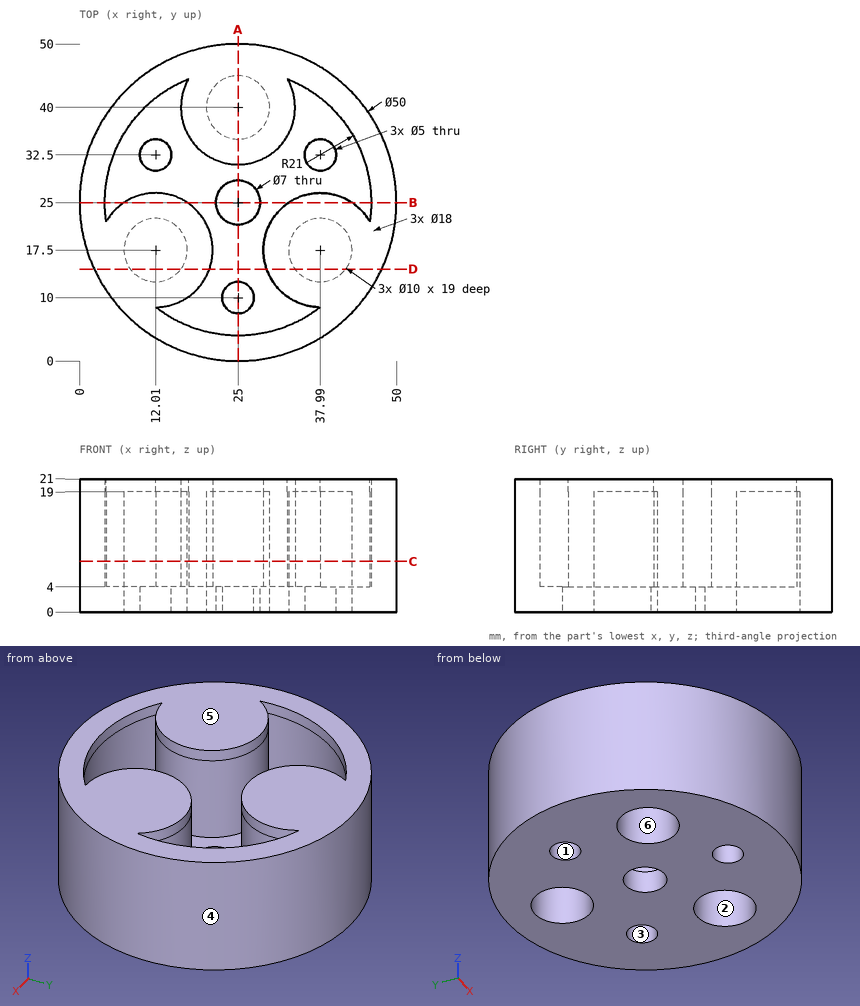
Check sheet for the drawn part. Datum: minimum x, y, z corner. Units: mm. A direction names the side the tool comes from. Coordinates: 2 decimals unless noted, no trailing zeros. Loops run counter-clockwise (first coordinate to the right, second up) from the corner with the lowest first, then second, coordinate; pieces in that order, holes last. Notation, with made-up numbers: (21, 38) -> (56, 38) arc R22 cw to (56, 55) -> close; hole circle Ø10 at (61, -6.75). An arc over 180 degrees is marked (long way). Answer in a Markdown table with one row per item.
1) Section check A-A (x = 25). Record the cut outline in (y, z).
The answers:
| item | result |
|---|---|
| outline | (0, 0) -> (7.5, 0) -> (7.5, 4) -> (4, 4) -> (4, 21) -> (0, 21) -> close; (12.5, 0) -> (21.5, 0) -> (21.5, 4) -> (12.5, 4) -> close; (28.5, 0) -> (35, 0) -> (35, 19) -> (45, 19) -> (45, 0) -> (50, 0) -> (50, 21) -> (31, 21) -> (31, 4) -> (28.5, 4) -> close |
2) Section check C-C (z = 8). Record the cut outline in (x, y) (1 decimal).
The answers:
| item | result |
|---|---|
| outline | circle Ø50 at (25, 25); hole (4.2, 22) arc R9 cw (long way) to (12, 8.5) arc R21 ccw to (38, 8.5) arc R9 cw (long way) to (45.8, 22) arc R21 ccw to (32.8, 44.5) arc R9 cw (long way) to (17.2, 44.5) arc R21 ccw to start; hole circle Ø10 at (12, 17.5); hole circle Ø10 at (25, 40); hole circle Ø10 at (38, 17.5) |
3) Access from +Z, -Z, +X, -X, +Y, -Y to the whole of each face (thin tool, end or side, straight path). Record for the marked faces 1 and 2.
The answers:
| item | result |
|---|---|
| face 1 | +Z, -Z |
| face 2 | -Z |
4) Draft check along X on the marked faces 3, 4, 5 and 6. Enter one of: released by +X, released by -X, zero draft, split by the parting line, or undercut.
The answers:
| item | result |
|---|---|
| face 3 | undercut |
| face 4 | split by the parting line |
| face 5 | zero draft |
| face 6 | undercut |
5) Scan lines: line 1 along Y through (x, z) = (25, 1); line 2 along X through (y, z) = (32.5, 2.5); line 3 along Y through (x, z) = (30.5, 16.75) (1 decimal). Record each from-to range of solid material in increasing order. Write a range as from..to.
The answers:
| item | result |
|---|---|
| line 1 | y = 0..7.5, 12.5..21.5, 28.5..35, 45..50 |
| line 2 | x = 1.15..9.51, 14.51..35.49, 40.49..48.85 |
| line 3 | y = 0.6..4.7, 12.5..22.5, 32.9..49.4 |
6) Section check B-B (y = 25). Record the cut outline in (x, z) (1 decimal), and give its area (3 significant figures).
The answers:
| item | result |
|---|---|
| outline | (0, 0) -> (21.5, 0) -> (21.5, 4) -> (17, 4) -> (17, 21) -> (7, 21) -> (7, 4) -> (4, 4) -> (4, 21) -> (0, 21) -> close; (28.5, 0) -> (50, 0) -> (50, 21) -> (46, 21) -> (46, 4) -> (43, 4) -> (43, 21) -> (33, 21) -> (33, 4) -> (28.5, 4) -> close |
| area | 646 mm2 |
7) Section check D-D (y = 14.5). Record the cut outline in (x, z) (1 decimal), and give its area (3 significant figures).
The answers:
| item | result |
|---|---|
| outline | (2.3, 0) -> (8, 0) -> (8, 19) -> (16, 19) -> (16, 0) -> (34, 0) -> (34, 19) -> (42, 19) -> (42, 0) -> (47.7, 0) -> (47.7, 21) -> (29.5, 21) -> (29.5, 4) -> (20.5, 4) -> (20.5, 21) -> (2.3, 21) -> close |
| area | 496 mm2 |
8) Depth check by flat-ended pin: P1, Ø6, axis at x = 12.01, y = 32.5, coming from the +Z side; P2, Ø3, axis at x = 40, y = 19.5, coming from the -Z side; P3, Ø1.5, axis at x = 19, z = 5, coming from the -Y side; P4, Ø3, axis at x = 25, y = 10, coming from the +Z side. Enter the tip coordinate at first touch or a pass-through.
The answers:
| item | result |
|---|---|
| P1 | stops at z = 4 |
| P2 | stops at z = 19 |
| P3 | stops at y = 0.56 |
| P4 | passes through |
